Answer from the drawing. Dimensions are ordinates in mm from the lowest x, y and z of the part. A direction names the side the tool comes from. Give positions to 0.01 mm unless a question says otherwise; leave off trailing zeros. Write each loop counter-clockwise with the first axis right and the second up, starting at its lowest first coordinate (ties: lowest second). Pieces come first, ordered by that corner, then holes.
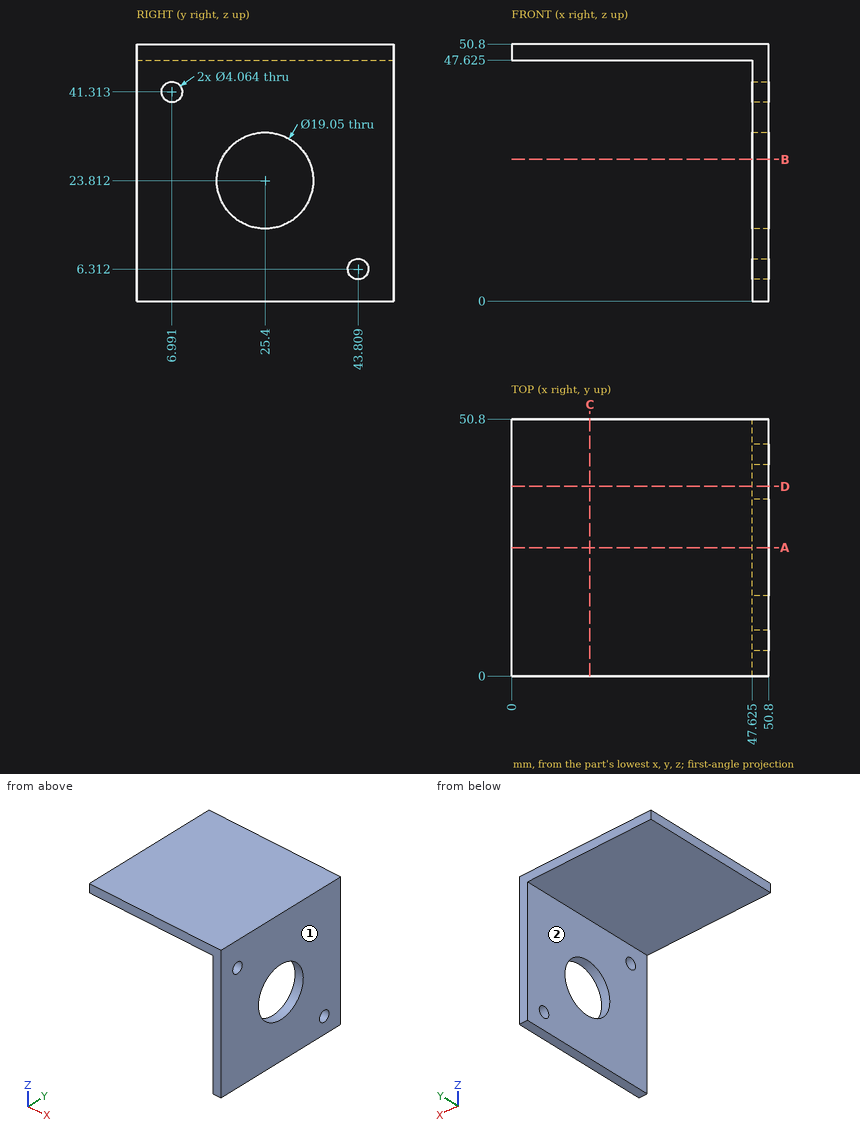
Item 1: A cutting plane is placed at C-C, the plane x = 15.5. Give the vertices of the cut face in (y, z) (1 decimal), plus the area to 3 significant figures.
Conclusion:
outline: (0, 47.6) - (50.8, 47.6) - (50.8, 50.8) - (0, 50.8) - close
area: 161 mm2
Item 2: A cutting plane is placed at A-A, the plane y = 25.4. Give the vertices of the cut face in (x, z) (1 decimal).
Conclusion:
outline: (0, 47.6) - (47.6, 47.6) - (47.6, 33.3) - (50.8, 33.3) - (50.8, 50.8) - (0, 50.8) - close; (47.6, 0) - (50.8, 0) - (50.8, 14.3) - (47.6, 14.3) - close
Item 3: Each of these flat-tipped pins is pushed along its axis until it touches: P1, Ø24, axis at y = 21.5, z = 13.5, coming from the -X side (1 decimal); P2, Ø3.5, axis at y = 6.99, z = 41.31, coming from the +X side; P3, Ø12, axis at y = 24.5, z = 27.5, coming from the +X side. Where does it stop, or does it pass through?
Conclusion:
P1: stops at x = 47.6
P2: passes through
P3: stops at x = 50.8
Item 4: A cutting plane is placed at B-B, the plane z = 28. Give the vertices of the cut face in (x, y) (1 decimal), plus the area to 3 significant figures.
Conclusion:
outline: (47.6, 0) - (50.8, 0) - (50.8, 16.8) - (47.6, 16.8) - close; (47.6, 34) - (50.8, 34) - (50.8, 50.8) - (47.6, 50.8) - close
area: 107 mm2
Item 5: A cutting plane is placed at D-D, the plane y = 37.5. Give the vertices of the cut face in (x, z) (1 decimal).
Conclusion:
outline: (0, 47.6) - (47.6, 47.6) - (47.6, 0) - (50.8, 0) - (50.8, 50.8) - (0, 50.8) - close
Item 6: Consider probe 1 along Z at (x, y) = (48, 25) (1 decimal); probe 2 along Z at (x, y) = (12.5, 4.5) (1 decimal). Determine where each line is inside the solid, lowest interval first.
Conclusion:
probe 1: z = 0 to 14.3, 33.3 to 50.8
probe 2: z = 47.6 to 50.8
Item 7: Which of the six approach directions +Z, -Z, +X, -X, +Y, -Y give full straight-line access (tool end or side, diameter ignored) to the marked faces 1 and 2?
Conclusion:
face 1: +Z, -Z, +X, +Y, -Y
face 2: -Z, -X, +Y, -Y
